CAD build for the part. Positions are in the model's coordinates, mm. Face numbers are marked on the shaded views. A direction names the side the tool comes from. Coordinates: 2 decimals unless noted, no trailing zeros. Order: outer loops, then holes, each group sorted by start corner. A loop starts at its lowest first (then second) coordinate and runs counter-clockwise, first axis right, second up. Notation, with made-up numbers: (-10, 18) - (14, 18) arc R19 cw to (14, 52) - close; hole circle Ø1 at (48, -40). An arc over 180 degrees is marked (long way). Return JSON: item names as keys, results as strings.
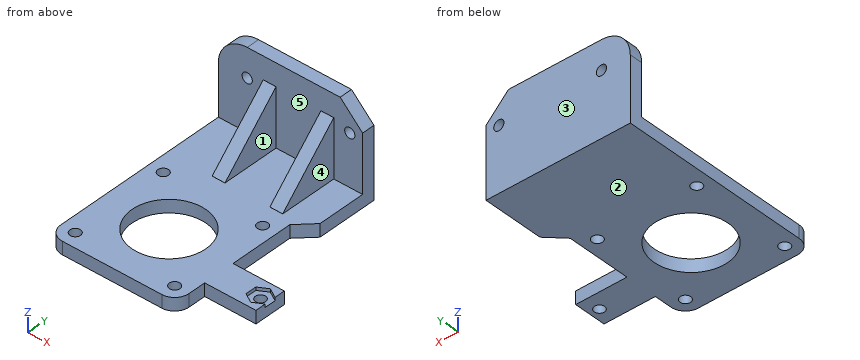
from build123d import *

# Parameters (mm, degrees)
PAD001_DEPTH      = 25
PAD001_DEPTH_BACK = 20
SKETCH002_W       = 4
SKETCH002_H       = 18
PAD002_DEPTH      = 22
SKETCH003_R       = 1.6
POCKET_DEPTH      = 44.001
FILLET001_R       = 9
CHAMFER_SIZE      = 7
CHAMFER001_SIZE   = 5
CHAMFER002_SIZE   = 17.99
SKETCH004_W       = 16
SKETCH004_H       = 10
PAD003_DEPTH      = 4
SKETCH005_R       = 1.6
POCKET001_DEPTH   = 4.001
POCKET002_DEPTH   = 1.5
SKETCH_W          = 40
SKETCH_H          = 40
SKETCH_R          = 1.65
SKETCH_R_2        = 11.5
PAD_DEPTH         = 4
FILLET_R          = 4.5


with BuildPart() as clippingbody:
    # Sketch001 → Pad001 (new body, two sides)
    with BuildSketch(Plane.YZ) as pad001_sk:
        Polygon((20, 0), (44, 0), (44, 29), (40, 29), (40, 4), (20, 4), align=None)
    extrude(amount=PAD001_DEPTH)
    extrude(pad001_sk.sketch, amount=-PAD001_DEPTH_BACK)

    # Sketch002 → Pad002 (join)
    with BuildSketch(Plane.XY):
        with Locations((14, 31)):
            Rectangle(SKETCH002_W, SKETCH002_H)
        with Locations((-4, 31)):
            Rectangle(SKETCH002_W, SKETCH002_H)
    extrude(amount=PAD002_DEPTH)

    # Sketch003 → Pocket (cut, through all)
    with BuildSketch(Plane.XZ):
        with Locations((21, 20)):
            Circle(SKETCH003_R)
        with Locations((-11, 20)):
            Circle(SKETCH003_R)
    extrude(amount=-POCKET_DEPTH, mode=Mode.SUBTRACT)

    # Fillet001
    fillet001_edges = [clippingbody.edges().sort_by_distance(p)[0] for p in [
        (-20, 42, 29),
    ]]
    fillet(fillet001_edges, radius=FILLET001_R)

    # Chamfer
    chamfer_edges = [clippingbody.edges().sort_by_distance(p)[0] for p in [
        (25, 42, 29),
    ]]
    chamfer(chamfer_edges, length=CHAMFER_SIZE)

    # Chamfer001
    chamfer001_edges = [clippingbody.edges().sort_by_distance(p)[0] for p in [
        (25, 20, 2),
    ]]
    chamfer(chamfer001_edges, length=CHAMFER001_SIZE)

    # Chamfer002
    chamfer002_edges = [clippingbody.edges().sort_by_distance(p)[0] for p in [
        (-4, 22, 22),
        (14, 22, 22),
    ]]
    chamfer(chamfer002_edges, length=CHAMFER002_SIZE)


with BuildPart() as sidestandbody:
    # Sketch004 → Pad003 (new body)
    with BuildSketch(Plane.XY):
        with Locations((28, -5)):
            Rectangle(SKETCH004_W, SKETCH004_H)
    extrude(amount=PAD003_DEPTH)

    # Sketch005 → Pocket001 (cut, through all)
    with BuildSketch(Plane.XY):
        with Locations((33, -5)):
            Circle(SKETCH005_R)
    extrude(amount=POCKET001_DEPTH, mode=Mode.SUBTRACT)

    # Sketch006 (on DatumPlane) → Pocket002 (cut)
    with BuildSketch(Plane.XY.offset(4.5)):
        Polygon((33, -8.464102), (36, -6.732051), (36, -3.267949), (33, -1.535898), (30, -3.267949), (30, -6.732051), align=None)
    extrude(amount=-POCKET002_DEPTH, mode=Mode.SUBTRACT)


with BuildPart() as holderfusion_refined:
    # Sketch → Pad (new body)
    with BuildSketch(Plane.XY):
        Rectangle(SKETCH_W, SKETCH_H)
        with Locations((-15.5, 15.5)):
            Circle(SKETCH_R, mode=Mode.SUBTRACT)
        with Locations((15.5, 15.5)):
            Circle(SKETCH_R, mode=Mode.SUBTRACT)
        with Locations((15.5, -15.5)):
            Circle(SKETCH_R, mode=Mode.SUBTRACT)
        with Locations((-15.5, -15.5)):
            Circle(SKETCH_R, mode=Mode.SUBTRACT)
        Circle(SKETCH_R_2, mode=Mode.SUBTRACT)
    extrude(amount=PAD_DEPTH)

    # Fillet
    fillet_edges = [holderfusion_refined.edges().sort_by_distance(p)[0] for p in [
        (20, -20, 2),
        (-20, -20, 2),
    ]]
    fillet(fillet_edges, radius=FILLET_R)

    # Fusion: union ClippingBody, SideStandBody
    add(clippingbody.part)
    add(sidestandbody.part)


solid = holderfusion_refined.part
Item 1: Which spindle directions (+Z, -Z, +X, -X, +Y, -Y) get a long thin tool onto all of the face, cutting with end or side? Do the marked faces 1 and 2. Say none if no direction does.
Findings below:
{"face 1": "+Z, -Y", "face 2": "-Z, +X, -X, +Y, -Y"}
Item 2: Band-saw the part on D-D, the plane x = 21. List the corners of the cut face in (y, z).
Findings below:
{"outline": "(-10, 0) - (0, 0) - (0, 4) - (-10, 4) - close; (21, 0) - (44, 0) - (44, 18.4) - (40, 18.4) - (40, 4) - (21, 4) - close; (40, 21.6) - (44, 21.6) - (44, 26) - (40, 26) - close"}
Item 3: Band-saw the part on A-A, the plane y = 26.5. List the corners of the cut face in (x, z), then the cut area to 3 significant figures.
Findings below:
{"outline": "(-20, 0) - (25, 0) - (25, 4) - (16, 4) - (16, 8.51) - (12, 8.51) - (12, 4) - (-2, 4) - (-2, 8.51) - (-6, 8.51) - (-6, 4) - (-20, 4) - close", "area": "216 mm²"}
Item 4: Band-saw the part on C-C, the plane z = 12. List the corners of the cut face in (x, y).
Findings below:
{"outline": "(-20, 40) - (-6, 40) - (-6, 29.99) - (-2, 29.99) - (-2, 40) - (12, 40) - (12, 29.99) - (16, 29.99) - (16, 40) - (25, 40) - (25, 44) - (-20, 44) - close"}
Item 5: Drop flat-ended pins along their axis: P1, Ø14.5, axis at y = 29, z = 11.5, coming from the -X side; P2, Ø3, axis at y = -14, z = 2, coming from the +X side; P3, Ø5.5, axis at y = 27, z = 15, coming from the +X side; P4, Ø2, axis at x = 26, z = 2.5, coming from the -Y side. Give the stop position or say it passes through.
Findings below:
{"P1": "stops at x = -6", "P2": "stops at x = 20", "P3": "passes through", "P4": "stops at y = -10"}
Item 6: Mould opens along X. For the marked faces 3, 4 and 5 say: released by +X, released by -X, zero draft, split by the parting line, or undercut.
Findings below:
{"face 3": "zero draft", "face 4": "released by +X", "face 5": "undercut"}
Item 7: Wall check: L1, parallel to Y at x = 15.5, z = 3; L2, parallel to Z at x = -11, y = 42.6; L3, parallel to Y at x = 33, z = 1.65. Give the ranges that are in metal, low to high. Write a range as [from, to].
Findings below:
{"L1": "y = [-20, -17.15], [-13.85, 13.85], [17.15, 44]", "L2": "z = [0, 18.4], [21.6, 29]", "L3": "y = [-10, -6.6], [-3.4, 0]"}
